Here's how the part is built. I have some questions about the finished solid (model axes, mm). A direction names the side the tool comes from. Round coordinates to 2 decimals unless told otherwise and drop trailing zeros. Loops run counter-clockwise (first coordinate to the right, second up) from the corner with the lowest first, then second, coordinate; pieces in that order, holes last. Notation, with made-up numbers: M 72.5,38 L 119.5,38 A17 ccw 119.5,55 Z; hole C 51,84.5 d10. An arc over 180 degrees is marked long. Answer as CSV lines item,"result".
```python
from build123d import *

# Parameters (mm, degrees)
PAD_DEPTH   = 20
THICKNESS_T = -1


with BuildPart() as part:
    # Sketch → Pad (new body)
    with BuildSketch(Plane.XY):
        with BuildLine():
            Line((-11.5, 14.25), (11.5, 14.25))
            ThreePointArc((16.5, 9.25), (15.035534, 12.785534), (11.5, 14.25))
            Line((16.5, 9.25), (16.5, -9.25))
            Line((16.5, -9.25), (-11.5, -9.25))
            Line((-11.5, -9.25), (-11.5, 14.25))
        make_face()
    extrude(amount=PAD_DEPTH)

    # Thickness
    thickness_openings = [part.faces().sort_by_distance(p)[0] for p in [
        (2.394093, 2.412589, 20),
    ]]
    offset(amount=THICKNESS_T, openings=thickness_openings)


solid = part.part
```
1. If I drill on line 1 (X direction, y = -0.25, z = 11); line 2 (Y direction, x = 6.5, z = 11.75), over which ranges is the centre line in solid material (lowest first)? Write a range as [from, to].
Evaluation:
line 1,"x = [-11.5, -10.5], [15.5, 16.5]"
line 2,"y = [-9.25, -8.25], [13.25, 14.25]"
2. We'd pull the mould along Y, two halves only. Please class faces 1 (the flat face through (15.5, 1, 10)), 2 (the flat face through (16.5, 0, 10)), 3 (the flat face through (3, 3, 1)), 4 (the flat face through (0, 14.25, 10)): pulls with the +Y half, pulls with the -Y half, needs draft (parallel to the pull), parting line crosses it, or undercut.
Evaluation:
face 1,"undercut"
face 2,"needs draft"
face 3,"undercut"
face 4,"pulls with the +Y half"
3. I want a section at C-C, the plane y = 3.5. Please give me the cut outline in (x, z), and give its area (3 significant figures).
Evaluation:
outline,"M -11.5,0 L 16.5,0 L 16.5,20 L 15.5,20 L 15.5,1 L -10.5,1 L -10.5,20 L -11.5,20 Z"
area,"66.0 mm²"
4. I want a section at B-B, the plane x = 8.5. Please give me the cut outline in (y, z).
Evaluation:
outline,"M -9.25,0 L 14.25,0 L 14.25,20 L 13.25,20 L 13.25,1 L -8.25,1 L -8.25,20 L -9.25,20 Z"
5. I want a section at A-A, the plane z = 3.5. Please give me the cut outline in (x, y), and give its area (3 significant figures).
Evaluation:
outline,"M -11.5,-9.25 L 16.5,-9.25 L 16.5,9.25 A5 ccw 11.5,14.25 L -11.5,14.25 Z; hole M -10.5,-8.25 L 15.5,-8.25 L 15.5,9.25 A4 ccw 11.5,13.25 L -10.5,13.25 Z"
area,"97.1 mm²"
6. Which directions (+Z, -Z, +X, -X, +Y, -Y) give clear straight access to the entire face, cutting with the end or side of a thin tool? Please do faces 5 (the cylindrical face through (14.359, 12.047, 10.367)), 6 (the flat face through (3, 3, 0)).
Evaluation:
face 5,"+Z"
face 6,"-Z, +X, -X, +Y, -Y"
7. For P1, Ø11, axis at x = -0.5, y = 5.5, coming from the +Z side, with a flat end and sliding along its axis, tell me the tip position at first contact or that it passes through.
Evaluation:
P1,"stops at z = 1"
